```python
from build123d import *

# Parameters (mm, degrees)
CUT_EXTRUDE_1_DEPTH = 1.3
FILLET_1_R          = 0.2
CHAMFER_1_SIZE      = 0.2


with BuildPart() as part:
    # 草图1 → 旋转1 (revolve)
    with BuildSketch(Plane.XY, mode=Mode.PRIVATE) as revolve_1_sk:
        Polygon((0, 0), (2.75, 0), (2.75, -2.93), (1.5, -2.93), (1.5, -22.93), (0, -22.93), align=None)
    revolve(revolve_1_sk.sketch.rotate(Axis((0, 0, 0), (0, -1, 0)), 90), axis=Axis((0, 0, 0), (0, -1, 0)))

    # 草图2 → 切除-拉伸1 (cut)
    with BuildSketch(Plane(origin=(0, 0, 0), x_dir=(1, 0, 0), z_dir=(0, 1, 0))):
        Polygon((0, 1.5), (-1.299038106, 0.75), (-1.299038106, -0.75), (0, -1.5), (1.299038106, -0.75), (1.299038106, 0.75), align=None)
    extrude(amount=-CUT_EXTRUDE_1_DEPTH, mode=Mode.SUBTRACT)

    # 圆角1
    fillet_1_edges = [part.edges().sort_by_distance(p)[0] for p in [
        (0, -2.93, -2.75),
        (0, 0, -2.75),
    ]]
    fillet(fillet_1_edges, radius=FILLET_1_R)

    # 倒角1
    chamfer_1_edges = [part.edges().sort_by_distance(p)[0] for p in [
        (0, -22.93, -1.5),
    ]]
    chamfer(chamfer_1_edges, length=CHAMFER_1_SIZE)


solid = part.part
```
Geometry check sheet. Reference: the model listing, model coordinates, mm. A direction names the side the tool comes from. Give positions to 0.01 mm unless a question says otherwise; leave off trailing zeros. Write each loop counter-clockwise with the first axis right and the second up, starting at its lowest first coordinate (ties: lowest second). Pieces come first, ordered by that corner, then holes. Notation, with made-up numbers: (-33, 10.25) - (-21, 10.25) arc R21 ccw to (-21, 20.25) - close; hole circle Ø11 at (13.25, 40). An arc over 180 degrees is marked (long way). Use a Markdown table: item, result.
Q1. Draft check along X on faces 3 (the face through (-0.45, -12.97, 1.43)), 4 (the face through (-1.299, -1, 0)), 5 (the face through (0, -2.93, 2)). Enter one of: pulls with the +X half, pulls with the -X half, needs draft (parallel to the pull), parting line crosses it, or undercut.
Computed:
| item | result |
|---|---|
| face 3 | parting line crosses it |
| face 4 | undercut |
| face 5 | needs draft |
Q2. Section check A-A, the plane z = 0. Enter the section's corners in (x, y), then the cut area to 3 significant figures.
Computed:
| item | result |
|---|---|
| outline | (-2.75, -2.73) arc R0.2 ccw to (-2.55, -2.93) - (-1.5, -2.93) - (-1.5, -22.73) - (-1.3, -22.93) - (1.3, -22.93) - (1.5, -22.73) - (1.5, -2.93) - (2.55, -2.93) arc R0.2 ccw to (2.75, -2.73) - (2.75, -0.2) arc R0.2 ccw to (2.55, 0) - (1.3, 0) - (1.3, -1.3) - (-1.3, -1.3) - (-1.3, 0) - (-2.55, 0) arc R0.2 ccw to (-2.75, -0.2) - close |
| area | 72.7 mm² |
Q3. Thickness scan on L1, parallel to X at y = -20.5, z = 0.1; L2, parallel to Y at x = -1.8, z = 0.05; L3, parallel to Y at x = 0.55, z = -0.7. Record the ranges inside material, lowest first. Write a range as [from, to].
Computed:
| item | result |
|---|---|
| L1 | x = [-1.5, 1.5] |
| L2 | y = [-2.93, 0] |
| L3 | y = [-22.93, -1.3] |
Q4. Go/stop test with flat-tipped pins: P1, Ø3, axis at x = -1, z = 1, coming from the -Y side; P2, Ø2, axis at y = -2.5, z = 2, coming from the -X side; P3, Ø3, axis at y = -7.5, z = 1, coming from the -X side; P4, Ø0.8, axis at x = 0, z = 0.5, coming from the +Y side. Record where each tip stops, or that it passes through.
Computed:
| item | result |
|---|---|
| P1 | stops at y = -22.93 |
| P2 | stops at x = -2.56 |
| P3 | stops at x = -1.5 |
| P4 | stops at y = -1.3 |
Q5. Section check B-B, the plane y = -13. Enter the section's corners in (x, z).
Computed:
| item | result |
|---|---|
| outline | circle Ø3 at (0, 0) |
Q6. Set-up check for faces 1 (the face through (0.64, -0.64, 1.13)), 2 (the face through (0, -22.93, 0)): record each of +Z, -Z, +X, -X, +Y, -Y from which the full face is reachable in a straight line by a thin tool's end or side.
Computed:
| item | result |
|---|---|
| face 1 | +Y |
| face 2 | +Z, -Z, +X, -X, -Y |
